from build123d import *

# Parameters (mm, degrees)
BOSS_EXTRUDE1_DEPTH = 2
FILLET1_R           = 2
SKETCH2_R           = 1.5
CUT_EXTRUDE1_DEPTH  = 10


with BuildPart() as part:
    # Sketch1 → Boss-Extrude1 (new body)
    with BuildSketch(Plane(origin=(0, 0, 0), x_dir=(1, 0, 0), z_dir=(0, 1, 0))):
        Polygon((-14, 33.798989873), (14, 33.798989873), (33.798989873, 14), (33.798989873, -14), (14, -33.798989873), (-14, -33.798989873), (-33.798989873, -14), (-33.798989873, 14), align=None)
    extrude(amount=BOSS_EXTRUDE1_DEPTH)

    # Fillet1
    fillet1_edges = [part.edges().sort_by_distance(p)[0] for p in [
        (-14, 1, -33.798989873),
        (14, 1, -33.798989873),
        (33.798989873, 1, -14),
        (33.798989873, 1, 14),
        (14, 1, 33.798989873),
        (-14, 1, 33.798989873),
        (-33.798989873, 1, 14),
        (-33.798989873, 1, -14),
    ]]
    fillet(fillet1_edges, radius=FILLET1_R)

    # Sketch2 → Cut-Extrude1 (cut)
    with BuildSketch(Plane(origin=(0, 2, 0), x_dir=(1, 0, 0), z_dir=(0, 1, 0))):
        with Locations(Location((-20, 20, 0), (0, 0, 270))):
            Circle(SKETCH2_R)
        with Locations(Location((20, 20, 0), (0, 0, 270))):
            Circle(SKETCH2_R)
        with Locations(Location((20, -20, 0), (0, 0, 270))):
            Circle(SKETCH2_R)
        with Locations(Location((-20, -20, 0), (0, 0, 270))):
            Circle(SKETCH2_R)
    extrude(amount=-CUT_EXTRUDE1_DEPTH, mode=Mode.SUBTRACT)


solid = part.part
Verification items for the finished model (mm, model axes). Round coordinates to 2 decimals unless told otherwise and drop trailing zeros. Order: outer loops, then holes, each group sorted by start corner. A loop starts at its lowest first (then second) coordinate and runs counter-clockwise, first axis right, second up. Notation, with made-up numbers: (-27.5, 7) -> (-12.5, 7) arc R18 ccw to (-12.5, 21) -> close; hole circle Ø8 at (-28.75, 69). An arc over 180 degrees is marked (long way). Put each result on its own line as item: value.
1) Section check C-C (x = -20). Record the cut outline in (y, z).
Final values:
outline: (0, -27.8) -> (2, -27.8) -> (2, -21.5) -> (0, -21.5) -> close; (0, -18.5) -> (2, -18.5) -> (2, 18.5) -> (0, 18.5) -> close; (0, 21.5) -> (2, 21.5) -> (2, 27.8) -> (0, 27.8) -> close
2) Section check B-B (z = -20). Record the cut outline in (x, y), then the cut area to 3 significant figures.
Final values:
outline: (-27.8, 0) -> (-21.5, 0) -> (-21.5, 2) -> (-27.8, 2) -> close; (-18.5, 0) -> (18.5, 0) -> (18.5, 2) -> (-18.5, 2) -> close; (21.5, 0) -> (27.8, 0) -> (27.8, 2) -> (21.5, 2) -> close
area: 99.2 mm^2
3) Mould release check, pull along Y, two halves, no side actions. Record for faces 1 (the flat face through (0, 2, 0)), 2 (the flat face through (0, 0, 0)), 3 (the flat face through (0, 1, 33.799)): +Y half, -Y half, draft (parallel to the pull), parting line (faces both ways), or undercut.
Final values:
face 1: +Y half
face 2: -Y half
face 3: draft
4) Section check D-D (x = 24). Record the cut outline in (y, z).
Final values:
outline: (0, -23.8) -> (2, -23.8) -> (2, 23.8) -> (0, 23.8) -> close
5) Section check A-A (y = 1.3). Record the cut outline in (x, z), then the cut area to 3 significant figures.
Final values:
outline: (-33.8, -13.17) arc R2 ccw to (-33.21, -14.59) -> (-14.59, -33.21) arc R2 ccw to (-13.17, -33.8) -> (13.17, -33.8) arc R2 ccw to (14.59, -33.21) -> (33.21, -14.59) arc R2 ccw to (33.8, -13.17) -> (33.8, 13.17) arc R2 ccw to (33.21, 14.59) -> (14.59, 33.21) arc R2 ccw to (13.17, 33.8) -> (-13.17, 33.8) arc R2 ccw to (-14.59, 33.21) -> (-33.21, 14.59) arc R2 ccw to (-33.8, 13.17) -> close; hole circle Ø3 at (-20, -20); hole circle Ø3 at (-20, 20); hole circle Ø3 at (20, -20); hole circle Ø3 at (20, 20)
area: 3,760 mm^2
6) Material ranges on line 1 (X direction, y = 1.3, z = -20); line 2 (Z direction, x = -15, y = 1.45); line 3 (Z direction, x = 15.5, y = 1.55), recorded low to high.
Final values:
line 1: x = -27.8 to -21.5, -18.5 to 18.5, 21.5 to 27.8
line 2: z = -32.8 to 32.8
line 3: z = -32.3 to 32.3
7) Depth check by flat-ended pin: pin 1 (3.5 mm diameter, centred on x = 20, z = 20, fed in from -Y); pin 2 (2.5 mm diameter, centred on x = -20, z = 20, fed in from +Y). Enter the tip coordinate at first touch or a pass-through.
Final values:
pin 1: stops at y = 0
pin 2: passes through
